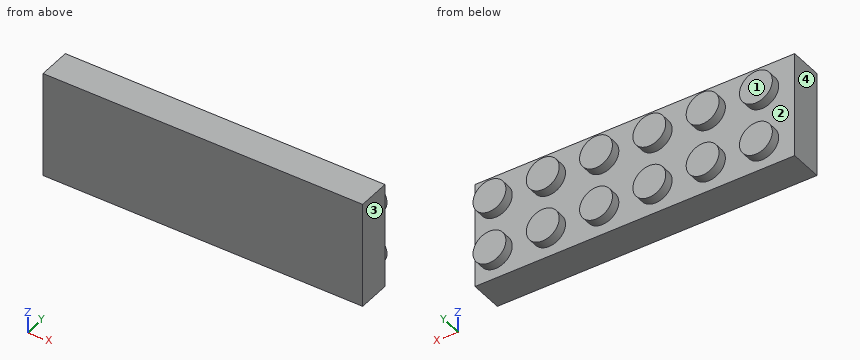
from build123d import *

# Parameters (mm, degrees)
F0_R     = 2.46
F1_DEPTH = 4.92
F2_R     = 2.46
F4_DEPTH = 1.4


# Not quite as in the source:
# - the program builds the solid bodies; features that only make, move or delete a surface that nothing else refers to are left out


with BuildPart() as f1:
    # F0 (on Front) → F1 (new body)
    with BuildSketch(Plane.XZ):
        Polygon((-47.81, 0), (0, 0), (0, 15.85), (-47.81, 15.85), (-47.81, 4.5985402539), align=None)
        with BuildLine():
            ThreePointArc((-42.89, 4.5985402539), (-45.35, 2.1385402539), (-47.81, 4.5985402539))
            ThreePointArc((-47.81, 4.5985402539), (-45.3923948453, 7.0581749173), (-42.8914612381, 4.6833173524))
            ThreePointArc((-42.8914612381, 4.6833173524), (-42.8903653367, 4.6409350993), (-42.89, 4.5985402539))
        make_face(mode=Mode.SUBTRACT)
        with BuildLine():
            ThreePointArc((-37.9729224851, 4.7680947078), (-40.3905275113, 2.3084600467), (-42.8914612381, 4.6833173524))
            ThreePointArc((-42.8914612381, 4.6833173524), (-40.475317459, 7.227729369), (-37.9729224851, 4.7680947078))
        make_face(mode=Mode.SUBTRACT)
        with Locations((-26.7290156335, 5.1733576693)):
            Circle(F0_R, mode=Mode.SUBTRACT)
        with Locations((-20.1186146587, 3.1614964828)):
            Circle(F0_R, mode=Mode.SUBTRACT)
        with Locations((-13.7956207618, 3.1614964828)):
            Circle(F0_R, mode=Mode.SUBTRACT)
        with BuildLine():
            ThreePointArc((-6.4156207618, 3.1614964828), (-8.8756207618, 0.7014964828), (-11.3356207618, 3.1614964828))
            ThreePointArc((-11.3356207618, 3.1614964828), (-8.8756207618, 5.6214964828), (-6.4156207618, 3.1614964828))
        make_face(mode=Mode.SUBTRACT)
        with Locations((-43.3987230062, 10.9215332195)):
            Circle(F0_R, mode=Mode.SUBTRACT)
        with Locations((-34.7764603794, 10.9215332195)):
            Circle(F0_R, mode=Mode.SUBTRACT)
        with BuildLine():
            ThreePointArc((-24.2718000183, 10.8045228756), (-29.1883194387, 10.9800549535), (-24.2690156335, 10.9215332195))
            ThreePointArc((-24.2690156335, 10.9215332195), (-24.2697118282, 10.8630114856), (-24.2718000183, 10.8045228756))
        make_face(mode=Mode.SUBTRACT)
        with BuildLine():
            ThreePointArc((-19.3545844044, 10.6875125042), (-21.8731061521, 8.2282086993), (-24.2718000183, 10.8045228756))
            ThreePointArc((-24.2718000183, 10.8045228756), (-21.7560626567, 13.1468163092), (-19.3545844044, 10.6875125042))
        make_face(mode=Mode.SUBTRACT)
        with Locations((-13.2208028808, 10.9215332195)):
            Circle(F0_R, mode=Mode.SUBTRACT)
        with Locations((-6.3229943626, 10.9215332195)):
            Circle(F0_R, mode=Mode.SUBTRACT)
        with BuildLine():
            ThreePointArc((-42.8914612381, 4.6833173524), (-45.3923948453, 7.0581749173), (-47.81, 4.5985402539))
            ThreePointArc((-47.81, 4.5985402539), (-45.35, 2.1385402539), (-42.89, 4.5985402539))
            ThreePointArc((-42.89, 4.5985402539), (-42.8903653367, 4.6409350993), (-42.8914612381, 4.6833173524))
        make_face()
        with BuildLine():
            ThreePointArc((-37.9729224851, 4.7680947078), (-40.475317459, 7.227729369), (-42.8914612381, 4.6833173524))
            ThreePointArc((-42.8914612381, 4.6833173524), (-40.3905275113, 2.3084600467), (-37.9729224851, 4.7680947078))
        make_face()
        with Locations((-43.3987230062, 10.9215332195)):
            Circle(F0_R)
        with Locations((-26.7290156335, 5.1733576693)):
            Circle(F0_R)
        with BuildLine():
            ThreePointArc((-24.2718000183, 10.8045228756), (-24.2697118282, 10.8630114856), (-24.2690156335, 10.9215332195))
            ThreePointArc((-24.2690156335, 10.9215332195), (-29.1883194387, 10.9800549535), (-24.2718000183, 10.8045228756))
        make_face()
        with BuildLine():
            ThreePointArc((-19.3545844044, 10.6875125042), (-21.7560626567, 13.1468163092), (-24.2718000183, 10.8045228756))
            ThreePointArc((-24.2718000183, 10.8045228756), (-21.8731061521, 8.2282086993), (-19.3545844044, 10.6875125042))
        make_face()
        with Locations((-20.1186146587, 3.1614964828)):
            Circle(F0_R)
        with Locations((-13.7956207618, 3.1614964828)):
            Circle(F0_R)
        with BuildLine():
            ThreePointArc((-6.4156207618, 3.1614964828), (-8.8756207618, 5.6214964828), (-11.3356207618, 3.1614964828))
            ThreePointArc((-11.3356207618, 3.1614964828), (-8.8756207618, 0.7014964828), (-6.4156207618, 3.1614964828))
        make_face()
        with Locations((-13.2208028808, 10.9215332195)):
            Circle(F0_R)
        with Locations((-6.3229943626, 10.9215332195)):
            Circle(F0_R)
        with Locations((-34.7764603794, 10.9215332195)):
            Circle(F0_R)
    extrude(amount=F1_DEPTH)

    # F2 (on Front) → F4 (join)
    with BuildSketch(Plane.XZ):
        with Locations((-42.9514177962, 11.845)):
            Circle(F2_R)
        with Locations((-42.9514177962, 3.875)):
            Circle(F2_R)
        with Locations((-34.9824780926, 11.975)):
            Circle(F2_R)
        with Locations((-34.9824780926, 4.005)):
            Circle(F2_R)
        with Locations((-27.0125882826, 11.9330903837)):
            Circle(F2_R)
        with Locations((-19.0425920932, 11.9408840209)):
            Circle(F2_R)
        with Locations((-11.0725940906, 3.9652414555)):
            Circle(F2_R)
        with Locations((-11.0725940906, 11.9352414555)):
            Circle(F2_R)
        with Locations((-3.1026442768, 3.9369577962)):
            Circle(F2_R)
        with Locations((-3.1026442768, 11.9069577962)):
            Circle(F2_R)
        with Locations((-19.0425920932, 3.9708840209)):
            Circle(F2_R)
        with Locations((-27.0125882826, 3.9630903837)):
            Circle(F2_R)
    extrude(amount=-F4_DEPTH)


solid = f1.part
Verification items for the finished model (mm, model axes). Face numbers are marked on the shaded views. Coordinates: 2 decimals unless noted, no trailing zeros. Loops run counter-clockwise (first coordinate to the right, second up) from the corner with the lowest first, then second, coordinate; pieces in that order, holes last. Notation, with made-up numbers: M 62.5,8.5 L 111.5,8.5 A24 ccw 111.5,36.5 Z; hole C -17,73.5 d3. An arc over 180 degrees is marked long. One line per item, written item: value.
1. Section check B-B on z = 13. Record the cut outline in (x, y), plus the area to 3 significant figures.
Answers follow:
outline: M -47.81,-4.92 L 0,-4.92 L 0,0 L -0.9,0 L -0.9,1.4 L -5.31,1.4 L -5.31,0 L -8.85,0 L -8.85,1.4 L -13.29,1.4 L -13.29,0 L -16.82,0 L -16.82,1.4 L -21.26,1.4 L -21.26,0 L -24.8,0 L -24.8,1.4 L -29.23,1.4 L -29.23,0 L -32.75,0 L -32.75,1.4 L -37.22,1.4 L -37.22,0 L -40.78,0 L -40.78,1.4 L -45.12,1.4 L -45.12,0 L -47.81,0 Z
area: 272 mm^2
2. Section check C-C on x = -29. Record the cut outline in (y, z), plus the area to 3 significant figures.
Answers follow:
outline: M -4.92,0 L 0,0 L 0,2.51 L 1.4,2.51 L 1.4,5.41 L 0,5.41 L 0,10.48 L 1.4,10.48 L 1.4,13.38 L 0,13.38 L 0,15.85 L -4.92,15.85 Z
area: 86.1 mm^2
3. Material ranges on line 1 along Y through (x, z) = (-11, 9); line 2 along X through (y, z) = (0.25, 14) (3 decimals); line 3 along X through (y, z) = (0.5, 13), recorded low to high. Write a range as from..to.
Answers follow:
line 1: -4.92..0
line 2: -44.138..-41.765, -36.379..-33.586, -28.347..-25.679, -20.389..-17.697, -12.41..-9.735, -4.395..-1.81
line 3: -45.12..-40.78, -37.22..-32.75, -29.23..-24.8, -21.26..-16.82, -13.29..-8.85, -5.31..-0.9
4. Mould release check, pull along X, two halves, no side actions. Record for the marked faces 1, 2, 3 and 4: pulls with the +X half, pulls with the -X half, needs draft (parallel to the pull), parting line crosses it, or undercut.
Answers follow:
face 1: needs draft
face 2: undercut
face 3: pulls with the +X half
face 4: pulls with the -X half
5. Section check A-A on y = 0.75. Give the number of separate pieces and of enclosed holes in the cut face, plus the area to 3 significant figures.
Answers follow:
separate pieces: 12
enclosed holes: 0
area: 228 mm^2
6. Section check D-D on x = -36.5. Record the cut outline in (y, z).
Answers follow:
outline: M -4.92,0 L 0,0 L 0,2.07 L 1.4,2.07 L 1.4,5.94 L 0,5.94 L 0,10.04 L 1.4,10.04 L 1.4,13.91 L 0,13.91 L 0,15.85 L -4.92,15.85 Z
